from build123d import *

# Parameters (mm, degrees)
SKETCH1_W           = 122
SKETCH1_H           = 112
BOSS_EXTRUDE1_DEPTH = 3
SKETCH3_R           = 2
CUT_EXTRUDE2_DEPTH  = 10
SKETCH4_R           = 1.25
CUT_EXTRUDE3_DEPTH  = 23
SKETCH5_R           = 1.25
CUT_EXTRUDE4_DEPTH  = 23
SKETCH6_R           = 1.65
SKETCH6_R_2         = 1.722739023
CUT_EXTRUDE5_DEPTH  = 10
SKETCH7_R           = 2.2
CUT_EXTRUDE6_DEPTH  = 10


with BuildPart() as part:
    # Sketch1 → Boss-Extrude1 (new body)
    with BuildSketch(Plane(origin=(0, 0, 0), x_dir=(1, 0, 0), z_dir=(0, 1, 0))):
        Rectangle(SKETCH1_W, SKETCH1_H)
    extrude(amount=BOSS_EXTRUDE1_DEPTH)

    # Sketch3 → Cut-Extrude2 (cut)
    with BuildSketch(Plane(origin=(0, 3, 0), x_dir=(1, 0, 0), z_dir=(0, 1, 0))):
        with Locations(Location((-53, 31, 0), (0, 0, 270))):
            Circle(SKETCH3_R)
        with Locations(Location((-53, 16, 0), (0, 0, 270))):
            Circle(SKETCH3_R)
        with Locations(Location((53, 16, 0), (0, 0, 270))):
            Circle(SKETCH3_R)
        with Locations(Location((53, 31, 0), (0, 0, 270))):
            Circle(SKETCH3_R)
    extrude(amount=-CUT_EXTRUDE2_DEPTH, mode=Mode.SUBTRACT)

    # Sketch4 → Cut-Extrude3 (cut)
    with BuildSketch(Plane(origin=(0, 3, 0), x_dir=(1, 0, 0), z_dir=(0, 1, 0))):
        with Locations(Location((-18, 41, 0), (0, 0, 270))):
            Circle(SKETCH4_R)
        with Locations(Location((-18, 5, 0), (0, 0, 270))):
            Circle(SKETCH4_R)
        with Locations(Location((18, 5, 0), (0, 0, 270))):
            Circle(SKETCH4_R)
        with Locations(Location((18, 41, 0), (0, 0, 270))):
            Circle(SKETCH4_R)
    extrude(amount=-CUT_EXTRUDE3_DEPTH, mode=Mode.SUBTRACT)

    # Sketch5 → Cut-Extrude4 (cut)
    with BuildSketch(Plane(origin=(0, 3, 0), x_dir=(1, 0, 0), z_dir=(0, 1, 0))):
        with Locations(Location((-38.25, -27.5, 0), (0, 0, 270))):
            Circle(SKETCH5_R)
        with Locations(Location((-28.75, -19.5, 0), (0, 0, 270))):
            Circle(SKETCH5_R)
        with Locations(Location((-28.75, -35.5, 0), (0, 0, 270))):
            Circle(SKETCH5_R)
        with Locations(Location((-19.25, -27.5, 0), (0, 0, 270))):
            Circle(SKETCH5_R)
        with Locations(Location((38.25, -27.5, 0), (0, 0, 270))):
            Circle(SKETCH5_R)
        with Locations(Location((19.25, -27.5, 0), (0, 0, 270))):
            Circle(SKETCH5_R)
        with Locations(Location((28.75, -35.5, 0), (0, 0, 270))):
            Circle(SKETCH5_R)
        with Locations(Location((28.75, -19.5, 0), (0, 0, 270))):
            Circle(SKETCH5_R)
    extrude(amount=-CUT_EXTRUDE4_DEPTH, mode=Mode.SUBTRACT)

    # Sketch6 → Cut-Extrude5 (cut)
    with BuildSketch(Plane(origin=(0, 3, 0), x_dir=(1, 0, 0), z_dir=(0, 1, 0))):
        with Locations(Location((-32, 41, 0), (0, 0, 270))):
            Circle(SKETCH6_R)
        with Locations(Location((-32, 9, 0), (0, 0, 270))):
            Circle(SKETCH6_R_2)
        with Locations(Location((32, 9, 0), (0, 0, 270))):
            Circle(SKETCH6_R_2)
        with Locations(Location((32, 41, 0), (0, 0, 270))):
            Circle(SKETCH6_R)
    extrude(amount=-CUT_EXTRUDE5_DEPTH, mode=Mode.SUBTRACT)

    # Sketch7 → Cut-Extrude6 (cut)
    with BuildSketch(Plane(origin=(0, 3, 0), x_dir=(1, 0, 0), z_dir=(0, 1, 0))):
        with Locations(Location((-56, -46, 0), (0, 0, 270))):
            Circle(SKETCH7_R)
        with Locations(Location((-56, -36, 0), (0, 0, 270))):
            Circle(SKETCH7_R)
    cut_extrude6 = extrude(amount=-CUT_EXTRUDE6_DEPTH, mode=Mode.SUBTRACT)

    # Mirror1: Cut-Extrude6 across plane
    add(cut_extrude6.mirror(Plane(origin=(0, 0, 0), x_dir=(0, 0, 1), z_dir=(1, 0, 0))), mode=Mode.SUBTRACT)


solid = part.part
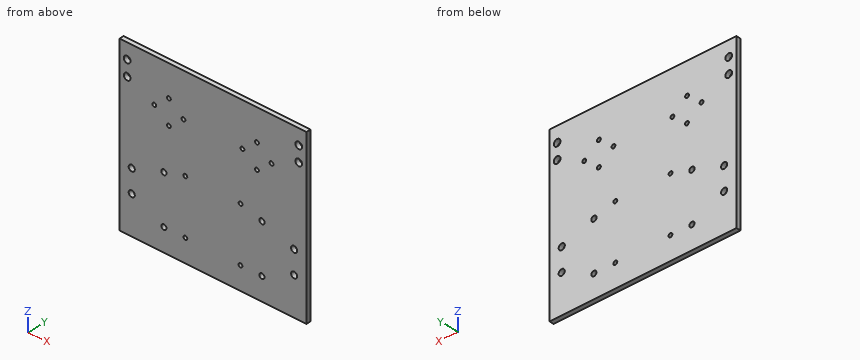
CAD build for the part. Positions are in the model's coordinates, mm. Coordinates: 2 decimals unless noted, no trailing zeros. Loops run counter-clockwise (first coordinate to the right, second up) from the corner with the lowest first, then second, coordinate; pieces in that order, holes last. Notation, with made-up numbers: (58.25, 67.5) - (70.25, 67.5) arc R22 ccw to (70.25, 106.5) - close; hole circle Ø7 at (86, 23.5). An arc over 180 degrees is marked (long way). Write item = value, one per line. Start each with the question number.
Q1. Cut at B-B, the plane y = 2.45. Give the number of separate pieces and of enclosed holes in the cut face, then the cut area to 3 significant figures.
Q2. Cut at C-C, the plane z = -31. List the corners of the cut face in (x, y), then the cut area to 3 significant figures.
Q3. Flat gauge pin, fed straight in: pin 1 Ø1.5 at (x, z) = (45.5, -7) entering from -Y. Where does the tip first touch, or does it go through?
Q4. Cut at A-A, the plane z = 46. List the corners of the cut face in (x, y), then the cut area to 3 significant figures.
Q5. Drill centre lines: L1, parallel to X at y = 2.3, z = 19.5; L2, parallel to X at y = 1.05, z = 27.5; L3, parallel to X at y = 1.5, z = -16. Where is each one in solid material? Low to high.
Computed:
q1.separate_pieces = 1
q1.enclosed_holes = 24
q1.area = 13,500 mm²
q2.outline = (-61, 0) - (-55, 0) - (-55, 3) - (-61, 3) - close; (-51, 0) - (51, 0) - (51, 3) - (-51, 3) - close; (55, 0) - (61, 0) - (61, 3) - (55, 3) - close
q2.area = 342 mm²
q3.pin_1 = 0
q4.outline = (-61, 0) - (-58.2, 0) - (-58.2, 3) - (-61, 3) - close; (-53.8, 0) - (53.8, 0) - (53.8, 3) - (-53.8, 3) - close; (58.2, 0) - (61, 0) - (61, 3) - (58.2, 3) - close
q4.area = 340 mm²
q5.L1 = -61 to -30, -27.5 to 27.5, 30 to 61
q5.L2 = -61 to -39.5, -37 to -20.5, -18 to 18, 20.5 to 37, 39.5 to 61
q5.L3 = -61 to -55, -51 to 51, 55 to 61
